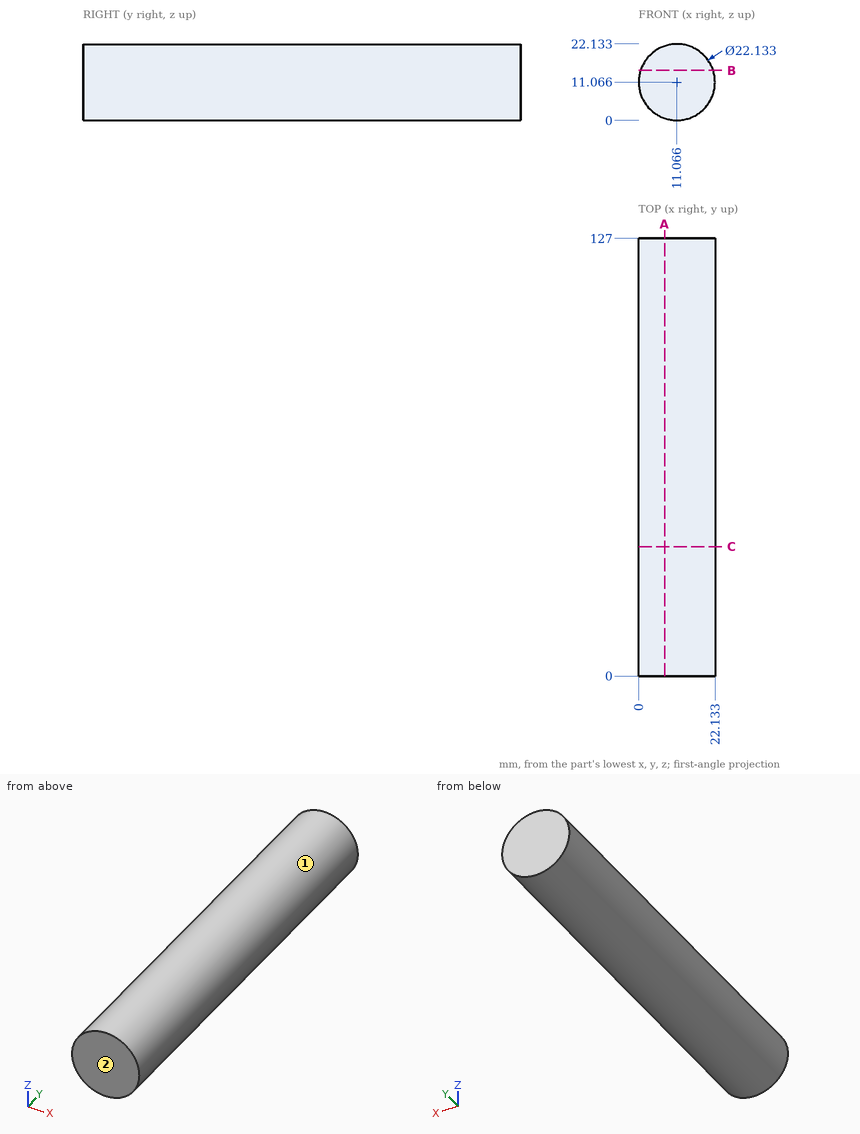
For this review, use the dimensioned drawing (mm, ordinates from the lowest corner) and the shaded views. Give positions to 0.01 mm unless a question says otherwise; leave off trailing zeros. Order: outer loops, then holes, each group sorted by start corner. A loop starts at its lowest first (then second) coordinate and runs counter-clockwise, first axis right, second up. Notation, with made-up numbers: (-31.75, 85.25) - (-7.75, 85.25) arc R19 cw to (-7.75, 116.25) - close; hole circle Ø7 at (-8, 38.5). An arc over 180 degrees is marked (long way). Use a Markdown table: item, result. Add a question column.
(1) Wall thickness on probe 1 along X at (y, z) = (56.5, 11.75); probe 2 along X at (y, z) = (84.5, 16); probe 3 along Z at (x, y) = (11.5, 98): over which ranges is each line inside the solid? List them lowest first. Write a range as [from, to].
(2) Clearance check with flat-ended pins moving along their axes: P1, Ø3, axis at x = 2.5, y = 111, coming from the +Z side; P2, Ø3, axis at y = 81.5, z = 13, coming from the +X side; P3, Ø8, axis at y = 83, z = 4.5, coming from the +X side. State where each tip first meets the part, or that it passes through.
(3) Mouldability with a two-part tool opening along X and no side actions: class the marked faces 1 and 2 as +X half, -X half, draft (parallel to the pull), parting line (faces both ways), or undercut.
(4) Add section A-A on x = 7.5. Give the boundary of the cut face in (y, z).
(5) Add section C-C on y = 37.5. Give the boundary of the cut face in (x, z), then the cut area to 3 significant figures.
(6) Add section B-B on z = 14.5. Give the boundary of the cut face in (x, y), then the cut area to 3 significant figures.
Report:
| question | item | result |
|---|---|---|
| 1 | probe 1 | x = [0.02, 22.11] |
| 1 | probe 2 | x = [1.16, 20.97] |
| 1 | probe 3 | z = [0.01, 22.12] |
| 2 | P1 | stops at z = 19.58 |
| 2 | P2 | stops at x = 22.12 |
| 2 | P3 | stops at x = 21.83 |
| 3 | face 1 | parting line |
| 3 | face 2 | draft |
| 4 | outline | (0, 0.59) - (127, 0.59) - (127, 21.54) - (0, 21.54) - close |
| 5 | outline | circle Ø22.13 at (11.07, 11.07) |
| 5 | area | 385 mm² |
| 6 | outline | (0.55, 0) - (21.59, 0) - (21.59, 127) - (0.55, 127) - close |
| 6 | area | 2,670 mm² |
